Autodesk Inventor part; units mm, degrees
ref_plane "YZ Plane" through (0, 0, 0) normal (1, 0, 0) x (0, 1, 0)
ref_plane "XZ Plane" through (0, 0, 0) normal (0, 1, 0) x (-1, 0, 0)
ref_plane "XY Plane" through (0, 0, 0) normal (0, 0, 1) x (1, 0, 0)
sketch "Sketch1" plane through (0, 0, 0) normal (0, 1, 0) x (-1, 0, 0)
  point P0 (0, 0)
sketch "Sketch2" plane through (0, 0, 0) normal (0, 1, 0) x (-1, 0, 0)
  line L0 (-76.2, 76.2) -> (76.2, 76.2)
  line L1 (76.2, 76.2) -> (76.2, -76.2)
  line L2 (76.2, -76.2) -> (-76.2, -76.2)
  line L3 (-76.2, -76.2) -> (-76.2, 76.2)
  line L4 (-76.2, 76.2) -> (76.2, -76.2) construction
  line L5 (76.2, 76.2) -> (-76.2, -76.2) construction
  point P0 (0, 0)
  dimension "d0" = 152.4
  dimension "d1" = 152.4
extrude "Extrusion1" add sketch "Sketch2" along normal blind 12.7
sketch "Sketch3" plane through (0, 12.7, 0) normal (0, 1, 0) x (1, 0, 0)
  line L0 (76.2, 76.2) -> (-76.2, 76.2)
  line L1 (76.2, -76.2) -> (76.2, 76.2)
  line L2 (-76.2, 76.2) -> (76.2, 76.2)
  line L3 (76.2, 76.2) -> (76.2, 63.5)
  line L4 (76.2, 63.5) -> (-76.2, 63.5)
  line L5 (-76.2, 63.5) -> (-76.2, 76.2)
  line L6 (-76.2, -76.2) -> (76.2, -76.2)
  line L7 (76.2, -76.2) -> (76.2, -63.5)
  line L8 (76.2, -63.5) -> (-76.2, -63.5)
  line L9 (-76.2, -63.5) -> (-76.2, -76.2)
  point P0 (0, 0)
  point P1 (76.2, -76.2)
  dimension "d4" = 12.7
  dimension "d5" = 12.7
  dimension "d15" = 152.4
extrude "Extrusion2" add sketch "Sketch3" along normal blind 127
fillet "Fillet1" radius 6.35 2 edges at (0, 0, 76.2) (0, 0, -76.2)
sketch "Sketch4" plane through (76.2, 12.7, -63.5) normal (1, 0, 0) x (0, 0, -1)
  circle A0 centre (-133.35, 57.15) radius 3.175
  circle A1 centre (6.35, 57.15) radius 3.175
  circle A2 centre (-63.5, -6.35) radius 3.175
  point P0 (-63.5, -12.7)
extrude "Extrusion3" cut sketch "Sketch4" against normal blind 12.7
sketch "Sketch5" plane through (-76.2, 12.7, 63.5) normal (-1, 0, 0) x (0, 0, 1)
  circle A0 centre (-133.35, 120.65) radius 3.175
  circle A1 centre (-133.35, 57.15) radius 3.175
  circle A2 centre (-133.35, 57.15) radius 3.175
  circle A3 centre (-133.35, -6.35) radius 3.175
  circle A4 centre (-63.5, -6.35) radius 3.175
  circle A5 centre (-63.5, -6.35) radius 3.175
  circle A6 centre (6.35, -6.35) radius 3.175
  circle A7 centre (6.35, 57.15) radius 3.175
  circle A8 centre (6.35, 57.15) radius 3.175
  circle A9 centre (6.35, 120.65) radius 3.175
  line L0 (6.35, -12.7) -> (-133.35, -12.7)
  point P0 (-63.5, -12.7)
  point P1 (-133.35, 120.65)
  point P2 (-133.35, -6.35)
  point P3 (6.35, -6.35)
  point P4 (6.35, 120.65)
  dimension "d20" = 69.85
sketch "Sketch6" plane through (0, 139.7, 0) normal (0, 1, 0) x (1, 0, 0)
  line L0 (76.2, 69.85) -> (-76.2, 69.85)
  circle A0 centre (0, 69.85) radius 3
  line L1 (-76.2, -69.85) -> (76.2, -69.85)
  circle A1 centre (0, -69.85) radius 3
  point P0 (0, 0)
  dimension "d16" = 6
  dimension "d17" = 6
extrude "Extrusion5" cut sketch "Sketch6" against normal blind 4
extrude "Extrusion6" cut sketch "Sketch5" against normal blind 12.7 contours A1 | A4 | A7
ref_plane "Work Plane1" through (76.2, 139.7, 76.2) normal (0.7071, -0.7071, 0) x (0, 0, -1)
sketch "Sketch7" plane through (76.2, 139.7, 76.2) normal (0.7071, -0.7071, 0) x (0, 0, -1)
  line L0 (139.7, 0) -> (152.4, 0)
  line L1 (146.05, 0) -> (146.05, -12.7)
  circle A0 centre (146.05, -12.7) radius 3.175
  line L2 (0, 0) -> (12.7, 0)
  line L3 (6.35, 0) -> (6.35, -12.7)
  circle A1 centre (6.35, -12.7) radius 3.175
  point P0 (76.2, -152.6644)
  dimension "d24" = 12.7
extrude "Extrusion7" cut sketch "Sketch7" along normal blind 31.75 and the other way blind 25.4
ref_plane "Work Plane2" through (76.2, 0, 76.2) normal (-0.7071, -0.7071, 0) x (0, 0, -1)
sketch "Sketch8" plane through (76.2, 0, 76.2) normal (-0.7071, -0.7071, 0) x (0, 0, -1)
  line L0 (6.35, 0) -> (146.05, 0)
  line L1 (146.05, 0) -> (146.05, -12.7)
  line L2 (146.05, 0) -> (146.05, -107.7631)
  line L3 (6.35, 0) -> (6.35, -12.7)
  line L4 (6.35, -107.7631) -> (6.35, 0)
  circle A0 centre (146.05, -12.7) radius 3.175
  circle A1 centre (6.35, -12.7) radius 3.175
  point P0 (76.2, -53.8815)
  dimension "d30" = 12.7
  dimension "d31" = 12.7
extrude "Extrusion8" cut sketch "Sketch8" along normal blind 25.4 and the other way blind 31.75
sketch "Sketch10" plane through (0, 12.7, 0) normal (0, 1, 0) x (1, 0, 0)
  line L0 (76.2, -63.5) -> (76.2, 63.5)
  line L1 (76.2, 0) -> (50.8, 0)
  circle A0 centre (50.8, 0) radius 2.6035
  line L2 (48.1965, 0) -> (-5.1435, 0)
  circle A1 centre (-7.747, 0) radius 2.6035
  line L3 (-5.1435, -17.8483) -> (-5.1435, 18.0947)
  line L4 (-5.1435, 0) -> (-5.1435, -49.2125)
  line L5 (23.8125, 0) -> (23.8125, -51.8414)
  line L6 (23.8125, 0) -> (23.8125, 51.8414)
  circle A2 centre (23.8125, -54.4449) radius 2.6035
  circle A3 centre (23.8125, 54.4449) radius 2.6035
  line L7 (30.1625, -51.8414) -> (15.875, -51.8414)
  line L8 (30.1625, 51.8414) -> (17.4625, 51.8414)
  point P0 (0, 0)
  dimension "d37" = 5.207
  dimension "d36" = 25.4
  dimension "d39" = 5.207
  dimension "d40" = 49.2125
  dimension "d41" = 51.8414
  dimension "d42" = 51.8414
  dimension "d43" = 5.207
extrude "Extrusion9" cut sketch "Sketch10" against normal blind 3.9878
sketch "Sketch11" plane through (0, 12.7, 0) normal (0, 1, 0) x (1, 0, 0)
  circle A0 centre (-7.747, 0) radius 2.6035
  line L0 (-10.3505, 29.2735) -> (-50.9905, 29.2735)
  line L1 (-63.5, -3.175) -> (-63.5, 3.175)
  line L2 (-50.8997, 16.5035) -> (-50.8997, 42.0435)
  circle A1 centre (-53.5032, 29.2735) radius 2.6035
  line L3 (-30.6705, 29.2735) -> (-30.6705, 2.6035)
  line L4 (-30.6705, 29.2735) -> (-30.6705, 55.9435)
  line L5 (-23.5267, 29.2578) -> (-40.9893, 29.2578)
  line L6 (-40.9893, 2.6035) -> (-17.4625, 2.6035)
  circle A2 centre (-30.6705, 0) radius 2.6035
  line L7 (-37.2049, 55.9435) -> (-23.5267, 55.9435)
  circle A3 centre (-30.6705, 58.547) radius 2.6035
  circle A4 centre (-7.747, 29.2578) radius 2.6035
  point P0 (0, 0)
  dimension "d46" = 40.64
  dimension "d47" = 5.207
  dimension "d48" = 26.67
  dimension "d49" = 26.67
  dimension "d59" = 5.207
  dimension "d60" = 5.207
  dimension "d61" = 5.207
extrude "Extrusion10" cut sketch "Sketch11" against normal blind 3.9878 contours A2 | A1 | A3 | A4
sketch "Sketch12" plane through (0, 12.7, 0) normal (0, 1, 0) x (1, 0, 0)
  point P0 (0, 0)
sketch "Sketch13" plane through (0, 12.7, 0) normal (0, 1, 0) x (1, 0, 0)
  circle A0 centre (-53.5032, 29.2735) radius 2.6035
  circle A1 centre (-30.6705, 0) radius 2.6035
  line L0 (-30.6705, -2.6035) -> (-30.6705, -38.1635)
  line L1 (-30.6705, -20.3835) -> (-43.3705, -20.3835)
  line L2 (-43.3705, -20.3835) -> (-17.9705, -20.3835)
  circle A2 centre (-45.974, -20.3835) radius 2.6035
  circle A3 centre (-15.367, -20.3835) radius 2.6035
  circle A4 centre (-30.6705, -40.767) radius 2.6035
  point P0 (0, 0)
  dimension "d65" = 5.207
  dimension "d66" = 5.207
  dimension "d67" = 5.207
  dimension "d62" = 35.56
  dimension "d63" = 12.7
  dimension "d64" = 25.4
extrude "Extrusion11" cut sketch "Sketch13" against normal blind 3.9878 contours A3 | A4 | A2
sketch "Sketch14" plane through (0, 12.7, 0) normal (0, 1, 0) x (1, 0, 0)
  line L0 (-76.2, -63.5) -> (76.2, -63.5)
  line L1 (-33.3375, -63.5) -> (-21.9075, -63.5)
  point P0 (0, 0)
properties part number "Fuselage_Body_Piece_Front"
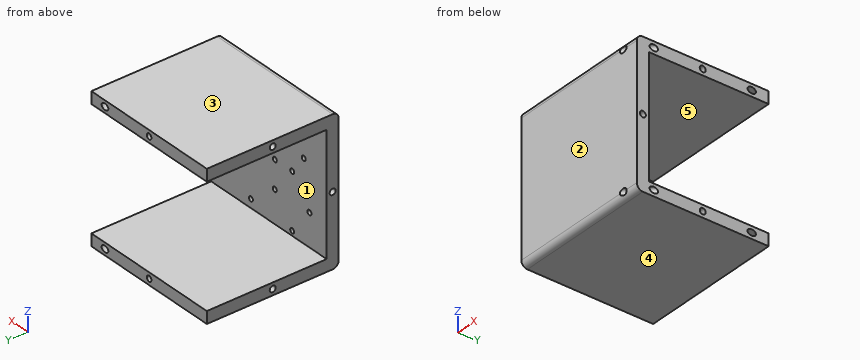
Build history of the part. All positions in model axes, mm. Face numbers are marked on the shaded views. A direction names the side the tool comes from. Round coordinates to 2 decimals unless told otherwise and drop trailing zeros. Write each loop counter-clockwise with the first axis right and the second up, starting at its lowest first coordinate (ties: lowest second). Pieces come first, ordered by that corner, then holes. Notation, with made-up numbers: (58.25, -16) -> (70.25, -16) arc R14 cw to (70.25, 10) -> close; hole circle Ø1 at (44.5, 5.25). An arc over 180 degrees is marked (long way). Write item = value, one per line.
(1) Two-plate mould, pull along Z, no slides. Class the marked faces 1, 2 and 3: pulls with the +Z half, pulls with the -Z half, needs draft (parallel to the pull), parting line crosses it, or undercut.
Answer:
face_1 = undercut
face_2 = needs draft
face_3 = pulls with the +Z half
(2) Probe L1, parallel to Z at x = 0, y = 138.35; L2, parallel to Z at x = -5, y = 61.5; L3, parallel to Z at x = 67, y = 7. List the from-to ranges inside material, lowest first.
Answer:
L1 = -76.2 to -72.85, -66.85 to -63.5, 63.5 to 66.85, 72.85 to 76.2
L2 = -76.2 to -63.5, 63.5 to 76.2
L3 = -76.2 to -72.77, -66.93 to -3.11, 3.11 to 66.93, 72.77 to 76.2
(3) Band-saw the part on B-B (x = 0). Give the cut face in (y, z).
Answer:
outline = (0, -69.85) arc R6.35 ccw to (6.35, -76.2) -> (139.7, -76.2) -> (139.7, -72.85) -> (135.7, -72.85) -> (135.7, -66.85) -> (139.7, -66.85) -> (139.7, -63.5) -> (12.7, -63.5) -> (12.7, 63.5) -> (139.7, 63.5) -> (139.7, 66.85) -> (135.7, 66.85) -> (135.7, 72.85) -> (139.7, 72.85) -> (139.7, 76.2) -> (6.35, 76.2) arc R6.35 ccw to (0, 69.85) -> close
(4) Tool access for the marked faces 4 and 5: list every direction of +Z, -Z, +X, -X, +Y, -Y with a clear straight run to the whole face (end or side of a thin tool).
Answer:
face_4 = -Z, +X, -X, +Y, -Y
face_5 = +X, -X, +Y
(5) Band-saw the part on D-D (z = 46). Give the cut face in (x, y).
Answer:
outline = (-76.2, 0) -> (76.2, 0) -> (76.2, 12.7) -> (-76.2, 12.7) -> close
(6) Band-saw the part on A-A (y = 69.85). Give the cut face in (x, z) (3 decimals), then the cut area to 3 significant figures.
Answer:
outline = (-76.2, -76.2) -> (76.2, -76.2) -> (76.2, -73.025) -> (63.5, -73.025) -> (63.5, -66.675) -> (76.2, -66.675) -> (76.2, -63.5) -> (-76.2, -63.5) -> (-76.2, -66.675) -> (-63.5, -66.675) -> (-63.5, -73.025) -> (-76.2, -73.025) -> close; (-76.2, 63.5) -> (76.2, 63.5) -> (76.2, 66.675) -> (63.5, 66.675) -> (63.5, 73.025) -> (76.2, 73.025) -> (76.2, 76.2) -> (-76.2, 76.2) -> (-76.2, 73.025) -> (-63.5, 73.025) -> (-63.5, 66.675) -> (-76.2, 66.675) -> close
area = 3,550 mm2
(7) Flat gauge pins, fed straight in: pin 1 (1.6 mm diameter, centred on x = -30, z = -0.5, fed in from +Y); pin 2 (1.8 mm diameter, centred on x = -0.5, z = 71, fed in from +Y); pin 3 (5.5 mm diameter, centred on x = -9, z = -28, fed in from +Y). Where does each tip first touch, or does it go through?
Answer:
pin_1 = 8.71
pin_2 = 135.7
pin_3 = 12.7
(8) Band-saw the part on C-C (y = 35.5). Give the cut face in (x, z), then the cut area to 3 significant figures.
Answer:
outline = (-76.2, -76.2) -> (76.2, -76.2) -> (76.2, -63.5) -> (-76.2, -63.5) -> close; (-76.2, 63.5) -> (76.2, 63.5) -> (76.2, 76.2) -> (-76.2, 76.2) -> close
area = 3,870 mm2
